Job drawing, mm, ordinate dimensions from the low corner. One solid piece. A direction names the side the tool comes from. Coordinates: 2 decimals unless noted, no trailing zeros. Write each loop counter-clockwise with the first axis right and the second up, starting at its lowest first coordinate (ties: lowest second). Pieces come first, ordered by that corner, then holes. Notation, with made-up numbers: (26, -37) - (47, -37) arc R14 cw to (47, -17) - close; hole circle Ø9 at (59.25, 74). An arc over 180 degrees is marked (long way). Put each result on its own line as item: value. Start each with the question number.
1. Drill centre lines: L1, parallel to Y at x = 0.5, z = 10; L2, parallel to X at y = 29.6, z = 10; L3, parallel to Z at x = 15, y = 29.85. Where is each one in solid material? Low to high. Write a range as from..to.
2. Drop a flat-ended pin along its axis: P1, Ø6, axis at y = 10, z = 12.5, coming from the +X side. Give the stop position or say it passes through.
3. Which spindle directions (+Z, -Z, +X, -X, +Y, -Y) get a long thin tool onto all of the face, cutting with end or side? Do the marked faces 1 and 2. Say none if no direction does.
4. Saw through at B-B, the plane y = 20. Write the cut outline in (x, z).
5. Saw through at A-A, the plane z = 10. Write the cut outline in (x, y), plus the area to 3 significant figures.
6. Saw through at C-C, the plane x = 15. Write the cut outline in (y, z), plus the area to 3 significant figures.
7. Saw through at D-D, the plane z = 14.5. Write the cut outline in (x, y).
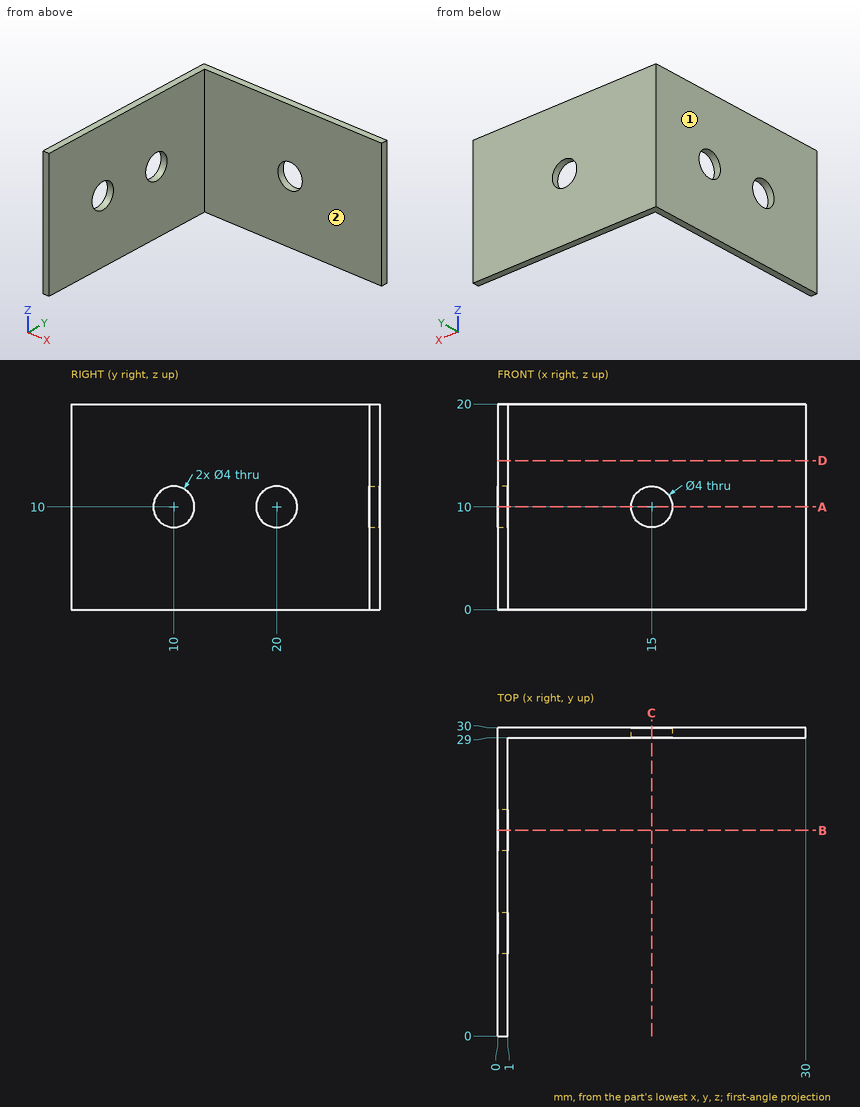
Final values:
1. L1: y = 0..8, 12..18, 22..30
1. L2: x = 0..13, 17..30
1. L3: z = 0..8, 12..20
2. P1: stops at x = 1
3. face 1: +Z, -Z, -X, +Y, -Y
3. face 2: +Z, -Z, +X, -Y
4. outline: (0, 0) - (1, 0) - (1, 8) - (0, 8) - close; (0, 12) - (1, 12) - (1, 20) - (0, 20) - close
5. outline: (0, 0) - (1, 0) - (1, 8) - (0, 8) - close; (0, 12) - (1, 12) - (1, 18) - (0, 18) - close; (0, 22) - (1, 22) - (1, 29) - (13, 29) - (13, 30) - (0, 30) - close; (17, 29) - (30, 29) - (30, 30) - (17, 30) - close
5. area: 47.0 mm²
6. outline: (29, 0) - (30, 0) - (30, 8) - (29, 8) - close; (29, 12) - (30, 12) - (30, 20) - (29, 20) - close
6. area: 16.0 mm²
7. outline: (0, 0) - (1, 0) - (1, 29) - (30, 29) - (30, 30) - (0, 30) - close
